Geometry check sheet. Reference: the model listing, model coordinates, mm. Give positions to 0.01 mm unless a question says otherwise; leave off trailing zeros. Write each loop counter-clockwise with the first axis right and the second up, starting at its lowest first coordinate (ties: lowest second). Pieces come first, ordered by that corner, then holes. Notation, with made-up numbers: (19.25, 42.5) - (46.25, 42.5) arc R31 ccw to (46.25, 76.5) - close; hole circle Ø1 at (23, 24.5). An arc over 180 degrees is marked (long way). Use a Markdown table: item, result.
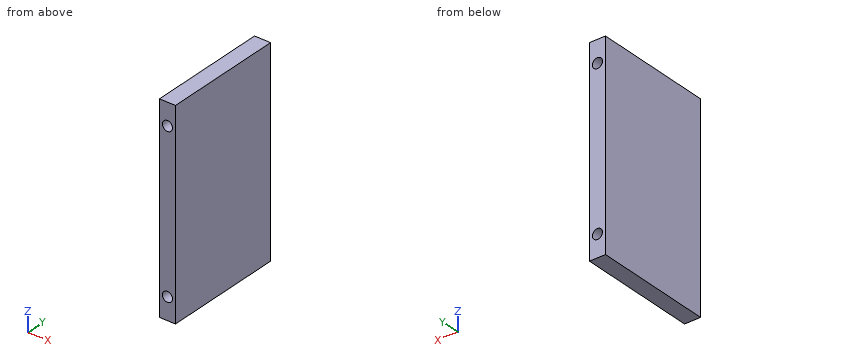
```python
from build123d import *

# Parameters (mm, degrees)
F0_W     = 76.2
F0_H     = 127
F1_DEPTH = 10.16
F2_R     = 3.175
F3_DEPTH = 6.35
F4_DEPTH = 6.35
F5_R     = 3.175
F6_DEPTH = 6.35


with BuildPart() as f1:
    # F0 (on Right) → F1 (new body)
    with BuildSketch(Plane.YZ):
        with Locations((-2.434241, 4.128012)):
            Rectangle(F0_W, F0_H)
    extrude(amount=F1_DEPTH)

    # F2 (on face) → F3 (cut)
    with BuildSketch(Plane.XZ.offset(40.534241)):
        with Locations((5.08, -45.528988)):
            Circle(F2_R)
    extrude(amount=-F3_DEPTH, mode=Mode.SUBTRACT)

    # F2 (on face) → F4 (cut)
    with BuildSketch(Plane.XZ.offset(40.534241)):
        with Locations((5.08, 53.785012)):
            Circle(F2_R)
    extrude(amount=-F4_DEPTH, mode=Mode.SUBTRACT)

    # F5 (on face) → F6 (cut)
    with BuildSketch(Plane(origin=(0, 35.665759, 0), x_dir=(-1, 0, 0), z_dir=(0, 1, 0))):
        with Locations((-5.08, 53.804278)):
            Circle(F5_R)
        with Locations((-5.08, -45.528988)):
            Circle(F5_R)
    extrude(amount=-F6_DEPTH, mode=Mode.SUBTRACT)


solid = f1.part
```
1) Section check A-A on x = 5.08. Record the boundary of the cut face in (y, z).
Working result:
| item | result |
|---|---|
| outline | (-40.53, -59.37) - (35.67, -59.37) - (35.67, -48.7) - (29.32, -48.7) - (29.32, -42.35) - (35.67, -42.35) - (35.67, 50.63) - (29.32, 50.63) - (29.32, 56.98) - (35.67, 56.98) - (35.67, 67.63) - (-40.53, 67.63) - (-40.53, 56.96) - (-34.18, 56.96) - (-34.18, 50.61) - (-40.53, 50.61) - (-40.53, -42.35) - (-34.18, -42.35) - (-34.18, -48.7) - (-40.53, -48.7) - close |
2) Depth check by flat-ended pin: P1, Ø1.9, axis at x = 6, z = 54, coming from the -Y side; P2, Ø1.9, axis at x = 6, z = -46.5, coming from the +Y side. Enter the tip coordinate at first touch or a pass-through.
Working result:
| item | result |
|---|---|
| P1 | stops at y = -34.18 |
| P2 | stops at y = 29.32 |
3) Material ranges on L1, parallel to Z at x = 5.08, y = -36.25; L2, parallel to Z at x = 7.75, y = 30; L3, parallel to Y at x = 6, z = -43, recorded low to high. Write a range as from..to.
Working result:
| item | result |
|---|---|
| L1 | z = -59.37..-48.7, -42.35..50.61, 56.96..67.63 |
| L2 | z = -59.37..-47.25, -43.81..52.09, 55.52..67.63 |
| L3 | y = -34.18..29.32 |
